```python
from build123d import *

# Parameters (mm, degrees)
ESQUISSE1_W        = 16
ESQUISSE1_H        = 16
BOSS_EXTRU_1_DEPTH = 0.9
ESQUISSE2_W        = 15
ESQUISSE2_H        = 15
BOSS_EXTRU_2_DEPTH = 2.3
ESQUISSE3_W        = 15.05
ESQUISSE3_H        = 15.05
BOSS_EXTRU_3_DEPTH = 4.65
ESQUISSE4_R        = 3
BOSS_EXTRU_4_DEPTH = 0.5
CONG_1_R           = 0.5
CONG_2_R           = 0.25


with BuildPart() as part:
    # Esquisse1 → Boss.-Extru.1 (new body)
    with BuildSketch(Plane(origin=(0, 0, 0), x_dir=(1, 0, 0), z_dir=(0, 1, 0))):
        Rectangle(ESQUISSE1_W, ESQUISSE1_H)
    extrude(amount=BOSS_EXTRU_1_DEPTH)

    # Esquisse2 → Boss.-Extru.2 (add)
    with BuildSketch(Plane(origin=(0, 0, 0), x_dir=(1, 0, 0), z_dir=(0, 1, 0))):
        Rectangle(ESQUISSE2_W, ESQUISSE2_H)
    extrude(amount=BOSS_EXTRU_2_DEPTH)

    # Esquisse3 → Boss.-Extru.3 (add)
    with BuildSketch(Plane(origin=(0, 2.3, 0), x_dir=(1, 0, 0), z_dir=(0, 1, 0))):
        Rectangle(ESQUISSE3_W, ESQUISSE3_H)
    extrude(amount=BOSS_EXTRU_3_DEPTH)

    # Esquisse4 → Boss.-Extru.4 (add)
    with BuildSketch(Plane(origin=(0, 6.95, 0), x_dir=(1, 0, 0), z_dir=(0, 1, 0))):
        with Locations(Location((0, 0, 0), (0, 0, 90))):
            Circle(ESQUISSE4_R)
    extrude(amount=BOSS_EXTRU_4_DEPTH)

    # Congé1
    cong_1_edges = [part.edges().sort_by_distance(p)[0] for p in [
        (0, 7.45, 3),
    ]]
    fillet(cong_1_edges, radius=CONG_1_R - 0.0001)  # a hair under: the kernel refuses the full size

    # Congé2
    cong_2_edges = [part.edges().sort_by_distance(p)[0] for p in [
        (7.525, 6.95, 0),
        (0, 6.95, -7.525),
        (-7.525, 6.95, 0),
        (0, 6.95, 7.525),
    ]]
    fillet(cong_2_edges, radius=CONG_2_R)


solid = part.part
```
Can you work these out from the model? Positions are in its coordinate system, mm. A direction names the side the tool comes from. Give positions to 0.01 mm unless a question says otherwise; leave off trailing zeros. Order: outer loops, then holes, each group sorted by start corner. A loop starts at its lowest first (then second) coordinate and runs counter-clockwise, first axis right, second up. Notation, with made-up numbers: M 33.5,-7.5 L 66.5,-7.5 A30 cw 66.5,19.5 Z; hole C -16.5,33 d5. An arc over 180 degrees is marked long. Write item = value, one per line. Start each with the question number.
Q1. For faces 1 (the flat face through (0, 4, 7.525)), 2 (the flat face through (-7.5, 2, 0)), 3 (the flat face through (7.525, 4, 0)), 4 (the flat face through (0, 2, -7.5)), 5 (the flat face through (-3.3, 6.95, -0.1)), which set-ups out of +Z, -Z, +X, -X, +Y, -Y let a thin tool reach every point of the face, with its end or its side?
Q2. We'd pull the mould along Y, two halves only. Please class faces 6 (the flat face through (0, 7.45, 0)), 7 (the flat face through (7.5, 2, 0)), 8 (the flat face through (8, 0.4, 0.1)): pulls with the +Y half, pulls with the -Y half, needs draft (parallel to the pull), parting line crosses it, or undercut.
Q3. Suppose I cut it at C-C (y = 5). Write out the boundary of the cut face in (x, z) (3 decimals), plus the area to 3 significant figures.
Q4. I need wall thicknesses on probe 1 along X at (y, z) = (4.75, -3) (3 decimals); probe 2 along Y at (x, z) = (-6.5, 3.5). Which ranges of each line are inside material? Lowest first, please. Write a range as [from, to].
Q5. Suppose I cut it at D-D (x = 4.25). Write out the boundary of the cut face in (y, z) (3 decimals).
Q6. Will these pins go through, and if not, where does the flat tip stop? pin 1 Ø2 at (x, y) = (0, 5) entering from +Z (3 decimals); pin 2 Ø3.5 at (y, z) = (4.5, 1.5) entering from -X (3 decimals); pin 3 Ø1 at (x, z) = (1, -2.5) entering from -Y; pin 4 Ø0.7 at (x, y) = (3, 1.5) entering from -Z.
Check result:
q1.face_1 = +Z, +X, -X, +Y
q1.face_2 = +Z, -Z, -X
q1.face_3 = +Z, -Z, +X, +Y
q1.face_4 = -Z, +X, -X
q1.face_5 = +Y
q2.face_6 = pulls with the +Y half
q2.face_7 = undercut
q2.face_8 = needs draft
q3.outline = M -7.525,-7.525 L 7.525,-7.525 L 7.525,7.525 L -7.525,7.525 Z
q3.area = 227 mm2
q4.probe_1 = [-7.525, 7.525]
q4.probe_2 = [0, 6.95]
q5.outline = M 0,-8 L 0.9,-8 L 0.9,-7.5 L 2.3,-7.5 L 2.3,-7.525 L 6.7,-7.525 A0.25 ccw 6.95,-7.275 L 6.95,7.275 A0.25 ccw 6.7,7.525 L 2.3,7.525 L 2.3,7.5 L 0.9,7.5 L 0.9,8 L 0,8 Z
q6.pin_1 = 7.525
q6.pin_2 = -7.525
q6.pin_3 = 0
q6.pin_4 = -7.5
